Build history of the part. All positions in model axes, mm. A direction names the side the tool comes from. Give positions to 0.01 mm unless a question says otherwise; leave off trailing zeros. Loops run counter-clockwise (first coordinate to the right, second up) from the corner with the lowest first, then second, coordinate; pieces in that order, holes last. Notation, with made-up numbers: (-5.5, 74) -> (47.5, 74) arc R19 cw to (47.5, 81) -> close; hole circle Ø4 at (-4, 57). An arc over 180 degrees is marked (long way). Answer as a JSON object with one key per item and string values. Group by question number.
Q1. Band-saw the part on B-B, the plane y = -6.5. Write the cut outline in (x, z), plus the area to 3 significant figures.
Q2. Band-saw the part on C-C, the plane z = 31. Write the cut outline in (x, y), plus the area to 3 significant figures.
Q3. Drop flat-ended pins along their axis: pin 1 (10 mm diameter, centred on x = -81, y = -10.5, fed in from +Z); pin 2 (5.5 mm diameter, centred on y = -7.5, z = 142.5, fed in from +X); pin 3 (4 mm diameter, centred on x = -54, y = -11.5, fed in from +Z). Give the stop position or say it passes through.
Q4. Band-saw the part on A-A, the plane z = 111. Write the cut outline in (x, y).
Q5. Tool access for faces 1 (the flat face through (426, -9, 129.345)), 2 (the flat face through (-158, -9, 129.345)), 3 (the flat face through (136, -17.78, 3)): list every direction of +Z, -Z, +X, -X, +Y, -Y with a clear straight run to the whole face (end or side of a thin tool).
Q6. Band-saw the part on D-D, the plane x = 211.5. Write the cut outline in (y, z).
Q7. Wall check: probe 1 along Z at (x, y) = (139.5, -11.25); probe 2 along X at (y, z) = (-1, 30); probe 3 along X at (y, z) = (-16.5, 34). Give the ranges that are in metal, low to high. Write a range as from..to.
from build123d import *

# Parameters (mm, degrees)
F1_DEPTH = 17.78


with BuildPart() as f1:
    # F0 (on Front) → F1 (new body)
    with BuildSketch(Plane.XZ):
        with BuildLine():
            ThreePointArc((413.79494, 147.127099), (291.400901, 41.730789), (134.39494, 3.812313))
            Line((134.39494, 3.812313), (134.39494, -26.667687))
            ThreePointArc((134.39494, -26.667687), (305.311948, 14.610443), (438.550347, 129.34508))
            Line((438.550347, 129.34508), (413.79494, 129.34508))
            Line((413.79494, 129.34508), (413.79494, 147.127099))
        make_face()
    extrude(amount=F1_DEPTH)

    # F2: F1 across face


with BuildPart() as f1_1:
    add(f1.part)
    add(f1.part.mirror(Plane(origin=(134.39494, -8.89, -11.427687), x_dir=(0, -1, 0), z_dir=(-1, 0, 0))))


solid = f1_1.part
Worked answers:
{
 "1": {"outline": "(-169.76, 129.35) arc R374.49 ccw to (134.39, -26.67) arc R374.49 ccw to (438.55, 129.35) -> (413.79, 129.35) -> (413.79, 147.13) arc R344.01 cw to (134.39, 3.81) arc R344.01 cw to (-145.01, 147.13) -> (-145.01, 129.35) -> close", "area": "20,300 mm2"},
 "2": {"outline": "(-65.27, -17.78) -> (0.36, -17.78) -> (0.36, 0) -> (-65.27, 0) -> close; (268.43, -17.78) -> (334.06, -17.78) -> (334.06, 0) -> (268.43, 0) -> close", "area": "2,330 mm2"},
 "3": {"pin 1": "z = 83.68", "pin 2": "x = 413.79", "pin 3": "z = 61.3"},
 "4": {"outline": "(-155.71, -17.78) -> (-115.12, -17.78) -> (-115.12, 0) -> (-155.71, 0) -> close; (383.91, -17.78) -> (424.49, -17.78) -> (424.49, 0) -> (383.91, 0) -> close"},
 "5": {"face 1": "+Z, +X, +Y, -Y", "face 2": "+Z, -X, +Y, -Y", "face 3": "+Z, -Z, +X, -X, -Y"},
 "6": {"outline": "(-17.78, -18.64) -> (0, -18.64) -> (0, 12.56) -> (-17.78, 12.56) -> close"},
 "7": {"probe 1": "-26.63..3.85", "probe 2": "-63.68..2.74, 266.05..332.47", "probe 3": "-69.95..-6.53, 275.31..338.74"}
}
